Build history of the part. All positions in model axes, mm. Coordinates: 2 decimals unless noted, no trailing zeros. Order: outer loops, then holes, each group sorted by start corner. A loop starts at its lowest first (then second) coordinate and runs counter-clockwise, first axis right, second up. Notation, with made-up numbers: (-24.5, 56) - (-7.5, 56) arc R10 ccw to (-7.5, 73) - close; hole circle Ø6 at (13.5, 18). An arc over 180 degrees is marked (long way). Write each question's results on one line, items separated by ' | '.
from build123d import *

# Parameters (mm, degrees)
SKETCH1_W           = 171.45
SKETCH1_H           = 63.5
SKETCH1_R           = 1.75
BOSS_EXTRUDE1_DEPTH = 4
CHAMFER1_SIZE       = 5
SKETCH3_W           = 3
SKETCH3_H           = 10.5
CUT_EXTRUDE2_DEPTH  = 4


with BuildPart() as part:
    # Sketch1 → Boss-Extrude1 (new body)
    with BuildSketch(Plane(origin=(0, 0, 0), x_dir=(1, 0, 0), z_dir=(0, 1, 0))):
        Rectangle(SKETCH1_W, SKETCH1_H)
        with Locations(Location((-76.2, 25.4, 0), (0, 0, 270))):
            Circle(SKETCH1_R, mode=Mode.SUBTRACT)
        with Locations(Location((-76.2, -25.4, 0), (0, 0, 270))):
            Circle(SKETCH1_R, mode=Mode.SUBTRACT)
        with Locations(Location((76.2, 25.4, 0), (0, 0, 270))):
            Circle(SKETCH1_R, mode=Mode.SUBTRACT)
        with Locations(Location((76.2, -25.4, 0), (0, 0, 270))):
            Circle(SKETCH1_R, mode=Mode.SUBTRACT)
    extrude(amount=BOSS_EXTRUDE1_DEPTH)

    # Chamfer1
    chamfer1_edges = [part.edges().sort_by_distance(p)[0] for p in [
        (85.725, 2, 31.75),
        (-85.725, 2, 31.75),
        (-85.725, 2, -31.75),
        (85.725, 2, -31.75),
    ]]
    chamfer(chamfer1_edges, length=CHAMFER1_SIZE)

    # Sketch3 → Cut-Extrude2 (cut)
    with BuildSketch(Plane(origin=(0, 4, 0), x_dir=(1, 0, 0), z_dir=(0, 1, 0))):
        with Locations((62, -26.5)):
            Rectangle(SKETCH3_W, SKETCH3_H)
        with Locations((62, 26.5)):
            Rectangle(SKETCH3_W, SKETCH3_H)
        with Locations((-62, -26.5)):
            Rectangle(SKETCH3_W, SKETCH3_H)
        with Locations((-62, 26.5)):
            Rectangle(SKETCH3_W, SKETCH3_H)
    extrude(amount=-CUT_EXTRUDE2_DEPTH, mode=Mode.SUBTRACT)


solid = part.part
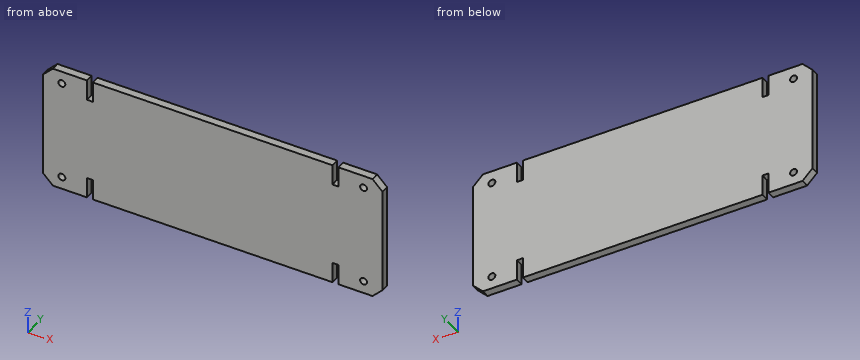
1. Band-saw the part on A-A on y = 1.2. Give the cut face in (x, z) (3 decimals).
Solved:
outline: (-85.725, -26.75) - (-80.725, -31.75) - (-63.5, -31.75) - (-63.5, -21.25) - (-60.5, -21.25) - (-60.5, -31.75) - (60.5, -31.75) - (60.5, -21.25) - (63.5, -21.25) - (63.5, -31.75) - (80.725, -31.75) - (85.725, -26.75) - (85.725, 26.75) - (80.725, 31.75) - (63.5, 31.75) - (63.5, 21.25) - (60.5, 21.25) - (60.5, 31.75) - (-60.5, 31.75) - (-60.5, 21.25) - (-63.5, 21.25) - (-63.5, 31.75) - (-80.725, 31.75) - (-85.725, 26.75) - close; hole circle Ø3.5 at (-76.2, -25.4); hole circle Ø3.5 at (-76.2, 25.4); hole circle Ø3.5 at (76.2, -25.4); hole circle Ø3.5 at (76.2, 25.4)
2. Probe line 1 (Z direction, x = 76.2, y = 2.8); line 2 (X direction, y = 1.2, z = 25.4) (3 decimals); line 3 (X direction, y = 0.55, z = 23) (3 decimals). List the from-to ranges inside material, lowest first.
Solved:
line 1: z = -31.75 to -27.15, -23.65 to 23.65, 27.15 to 31.75 | line 2: x = -85.725 to -77.95, -74.45 to -63.5, -60.5 to 60.5, 63.5 to 74.45, 77.95 to 85.725 | line 3: x = -85.725 to -63.5, -60.5 to 60.5, 63.5 to 85.725
3. Band-saw the part on B-B on x = -76.2. Give the cut face in (y, z), then the cut area to 3 significant figures.
Solved:
outline: (0, -31.75) - (4, -31.75) - (4, -27.15) - (0, -27.15) - close; (0, -23.65) - (4, -23.65) - (4, 23.65) - (0, 23.65) - close; (0, 27.15) - (4, 27.15) - (4, 31.75) - (0, 31.75) - close | area: 226 mm2
4. Drop a flat-ended pin along its axis: pin 1 Ø0.9 at (x, y) = (61.5, 3) entering from +Z. Give the stop position or say it passes through.
Solved:
pin 1: stops at z = 21.25
